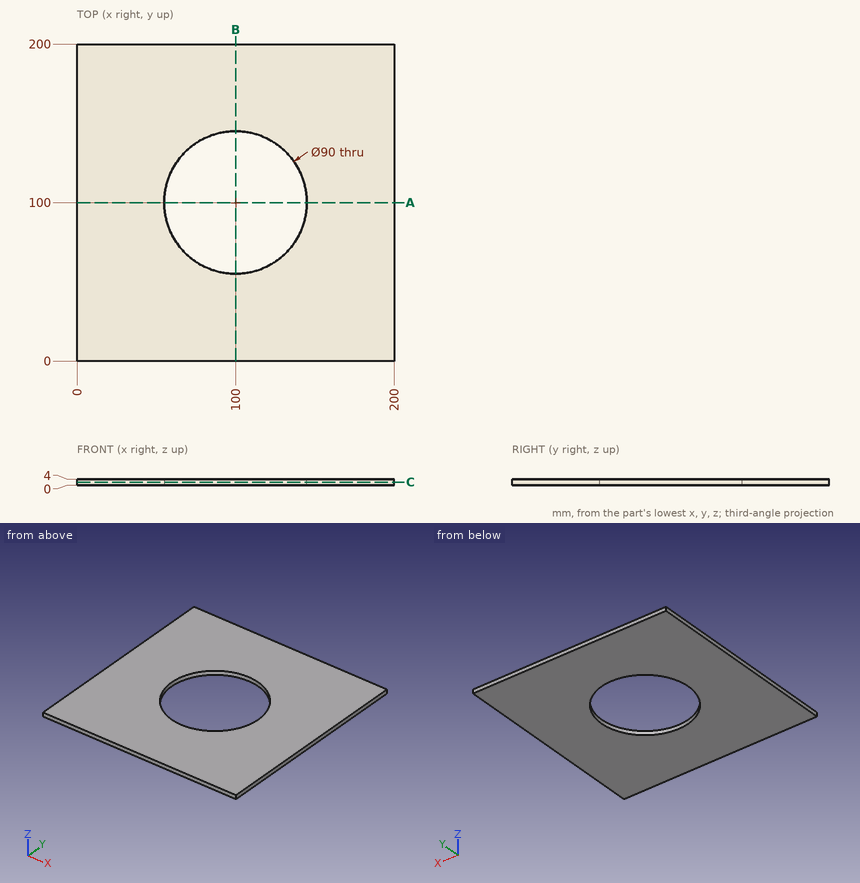
Design review of the part shown in the three views and the two pictorial views. Dimensions are in mm from the part's minimum x, y and z. Coordinates: 2 decimals unless noted, no trailing zeros. Loops run counter-clockwise (first coordinate to the right, second up) from the corner with the lowest first, then second, coordinate; pieces in that order, holes last.
Q1. We need section A-A on y = 100. State the section outline as (x, z) points, and give its area (3 significant figures).
Reported:
outline: (0, 0) - (55, 0) - (55, 4) - (0, 4) - close; (145, 0) - (200, 0) - (200, 4) - (145, 4) - close
area: 440 mm2
Q2. We need section C-C on z = 2. State the section outline as (x, y) points, and give its area (3 significant figures).
Reported:
outline: (0, 0) - (200, 0) - (200, 200) - (0, 200) - close; hole circle Ø90 at (100, 100)
area: 33,600 mm2
Q3. To check wall thickness, follow line 1 (Y direction, x = 100, z = 1.9); line 2 (X direction, y = 125, z = 0.3). State the ranges of each line that lie inside material, in increasing order.
Reported:
line 1: y = 0 to 55, 145 to 200
line 2: x = 0 to 62.58, 137.42 to 200
